```python
from build123d import *

# Parameters (mm, degrees)
SKETCH_1_R          = 4
EXTRUDE_1_DEPTH     = 10
HOLE_WIZARD_M10_1_D = 8.5
HOLE_WIZARD_M8_1_D  = 6.8


with BuildPart() as part:
    # 草图1 → 凸台-拉伸1 (new body)
    with BuildSketch(Plane.XY):
        with BuildLine():
            Line((125, -101), (125, 101))
            Line((125, 101), (-125, 101))
            Line((-125, 101), (-125, -101))
            Line((-125, -101), (-46, -101))
            Line((-46, -101), (-46, -55))
            ThreePointArc((-46, -55), (-44.535533906, -51.464466094), (-41, -50))
            Line((-41, -50), (41, -50))
            ThreePointArc((41, -50), (44.535533906, -51.464466094), (46, -55))
            Line((46, -55), (46, -101))
            Line((46, -101), (125, -101))
        make_face()
        with Locations((-85, -85)):
            Circle(SKETCH_1_R, mode=Mode.SUBTRACT)
        with Locations((85, -85)):
            Circle(SKETCH_1_R, mode=Mode.SUBTRACT)
        with Locations((-85, 85)):
            Circle(SKETCH_1_R, mode=Mode.SUBTRACT)
        with Locations((85, 85)):
            Circle(SKETCH_1_R, mode=Mode.SUBTRACT)
    extrude(amount=EXTRUDE_1_DEPTH)

    # M10 螺纹孔1 (through all)
    with Locations(Plane.XY.offset(10)):
        with Locations((85, -85), (-85, -85), (-85, 85), (85, 85)):
            Hole(HOLE_WIZARD_M10_1_D / 2)

    # M8 螺纹孔1 (through all)
    with Locations(Plane(origin=(0, 0, 0), x_dir=(-1, 0, 0), z_dir=(0, 0, -1))):
        with Locations((-50, 50), (0, 50), (50, 50), (-105, -81), (-65, -81), (65, -81), (105, -81)):
            Hole(HOLE_WIZARD_M8_1_D / 2)


solid = part.part
```
Verification items for the finished model (mm, model axes). A direction names the side the tool comes from. Coordinates: 2 decimals unless noted, no trailing zeros. Order: outer loops, then holes, each group sorted by start corner. A loop starts at its lowest first (then second) coordinate and runs counter-clockwise, first axis right, second up. Notation, with made-up numbers: (30.5, 47) - (75.5, 47) arc R26 ccw to (75.5, 85) - close; hole circle Ø5 at (-16, 72.5). An arc over 180 degrees is marked (long way). Return JSON: item names as keys, results as strings.
(1) Section check B-B, the plane x = -65. Record the cut outline in (y, z).
Filled sheet:
{"outline": "(-101, 0) - (-84.4, 0) - (-84.4, 10) - (-101, 10) - close; (-77.6, 0) - (101, 0) - (101, 10) - (-77.6, 10) - close"}
(2) Access from +Z, -Z, +X, -X, +Y, -Y to the whole of each face (thin tool, end or side, straight path). Record for faces 1 (the flat face through (-46, -78, 5)), 2 (the cylindrical face through (-107.698, -83.069, 5.07)).
Filled sheet:
{"face 1": "+Z, -Z, -Y", "face 2": "+Z, -Z"}
(3) Section check D-D, the plane y = -61. Record the cut outline in (x, z).
Filled sheet:
{"outline": "(-125, 0) - (-46, 0) - (-46, 10) - (-125, 10) - close; (46, 0) - (125, 0) - (125, 10) - (46, 10) - close"}
(4) Section check A-A, the plane y = 50. Record the cut outline in (x, z).
Filled sheet:
{"outline": "(-125, 0) - (-53.4, 0) - (-53.4, 10) - (-125, 10) - close; (-46.6, 0) - (-3.4, 0) - (-3.4, 10) - (-46.6, 10) - close; (3.4, 0) - (46.6, 0) - (46.6, 10) - (3.4, 10) - close; (53.4, 0) - (125, 0) - (125, 10) - (53.4, 10) - close"}
(5) Mould release check, pull along Y, two halves, no side actions. Record for faces 3 (the cylindrical face through (102.302, -83.069, 5.07)), 4 (the flat face through (2, 101, 5)), 5 (the flat face through (46, -78, 5)): pulls with the +Y half, pulls with the -Y half, needs draft (parallel to the pull), parting line crosses it, or undercut.
Filled sheet:
{"face 3": "undercut", "face 4": "pulls with the +Y half", "face 5": "needs draft"}
(6) Thickness scan on line 1 along Y through (x, z) = (85, 7); line 2 along Y through (x, z) = (0, 6); line 3 along Y through (x, z) = (50, 5.5). Record the ranges inside material, lowest first.
Filled sheet:
{"line 1": "y = -101 to -89.25, -80.75 to 80.75, 89.25 to 101", "line 2": "y = -50 to 46.6, 53.4 to 101", "line 3": "y = -101 to 46.6, 53.4 to 101"}
(7) Section check C-C, the plane z = 6.25. Give the number of separate pieces and of enclosed holes in the cut face, and give its area (3 significant figures).
Filled sheet:
{"separate pieces": "1", "enclosed holes": "11", "area": "45,300 mm^2"}
(8) Go/stop test with a flat-tipped pin: pin 1 (1.5 mm diameter, centred on x = 29.5, z = 7, fed in from -Y). Record where the tip stops, or that it passes through.
Filled sheet:
{"pin 1": "stops at y = -50"}
